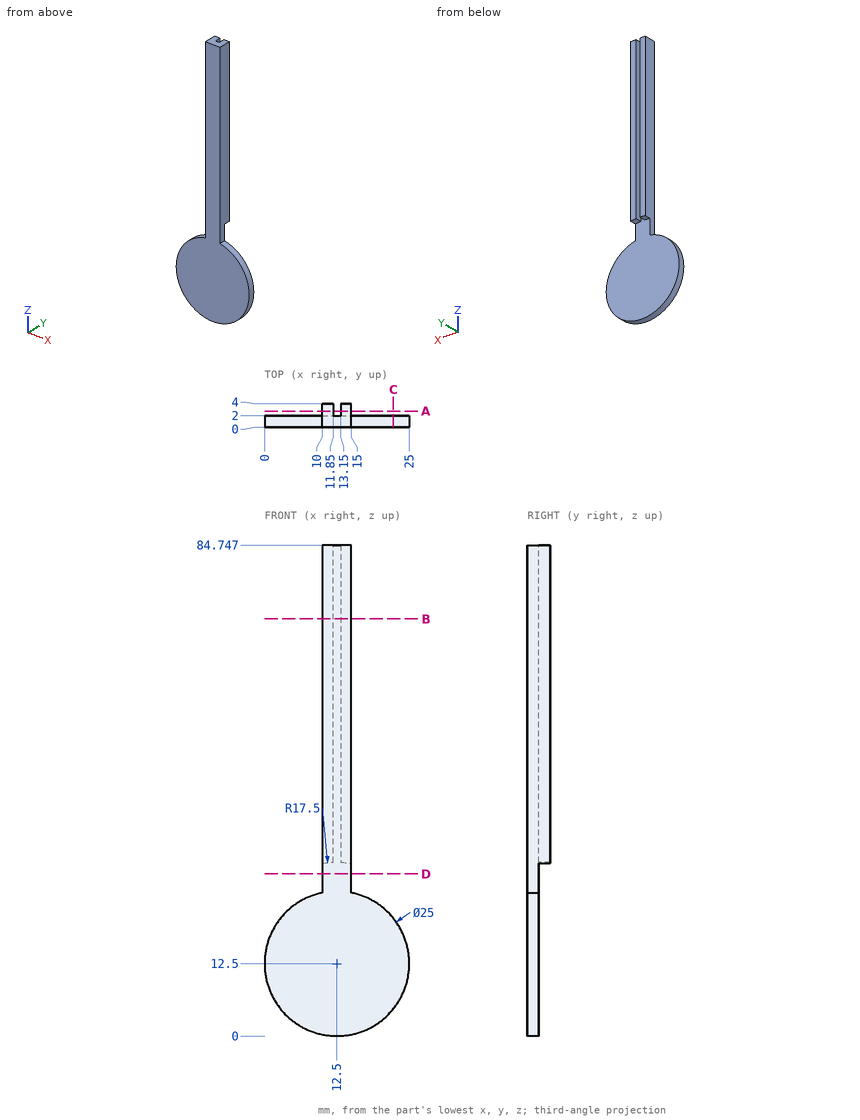
Study the drawing (mm; zero at the part's minimum x, y, z) and answer. Round coordinates to 2 decimals unless told otherwise and drop trailing zeros. Write each loop counter-clockwise with the first axis right and the second up, starting at its lowest first coordinate (ties: lowest second). Pieces come first, ordered by that corner, then holes. Notation, with made-up numbers: (-4.75, 79) - (18.25, 79) arc R29 cw to (18.25, 106) - close; hole circle Ø5 at (-27.75, 10). An arc over 180 degrees is marked (long way). Use a Markdown table: item, result. Add a question column.
1. The part is cut by section B-B (z = 72). Write down the section's boundary in (x, y).
2. Consider line 1 (X direction, y = 2.6, z = 69.5); line 2 (X direction, y = 0.65, z = 66.5); line 3 (Y direction, x = 13, z = 69). Determine where each line is inside the solid, lowest interval first.
3. The part is cut by section C-C (x = 22.25). Write down the section's boundary in (y, z), and give its area (3 significant figures).
4. The part is cut by section D-D (z = 28). Write down the section's boundary in (x, y), and give its area (3 significant figures).
5. Flat-ended cylindrical pins translate along their axes: P1, Ø1.2, axis at y = 1.5, z = 47.5, coming from the +X side; P2, Ø0.6, axis at y = 2.5, z = 66, coming from the -X side; P3, Ø10, axis at x = 20.5, z = 16, coming from the +Y side. Find the tip coordinate at first contact, or state that the pin passes through.
6. The part is cut by section A-A (y = 2.75). Write down the section's boundary in (x, z), and give its area (3 significant figures).
Reported:
| question | item | result |
|---|---|---|
| 1 | outline | (10, 0) - (15, 0) - (15, 4) - (13.15, 4) - (13.15, 2) - (11.85, 2) - (11.85, 4) - (10, 4) - close |
| 2 | line 1 | 10 to 11.85, 13.15 to 15 |
| 2 | line 2 | 10 to 15 |
| 2 | line 3 | 0 to 2 |
| 3 | outline | (0, 4.68) - (2, 4.68) - (2, 20.32) - (0, 20.32) - close |
| 3 | area | 31.3 mm^2 |
| 4 | outline | (10, 0) - (15, 0) - (15, 2) - (10, 2) - close |
| 4 | area | 10.0 mm^2 |
| 5 | P1 | x = 15 |
| 5 | P2 | x = 10 |
| 5 | P3 | y = 2 |
| 6 | outline | (10, 29.82) arc R17.5 cw to (11.85, 29.99) - (11.85, 84.75) - (10, 84.75) - close; (13.15, 29.99) arc R17.5 cw to (15, 29.82) - (15, 84.75) - (13.15, 84.75) - close |
| 6 | area | 203 mm^2 |
